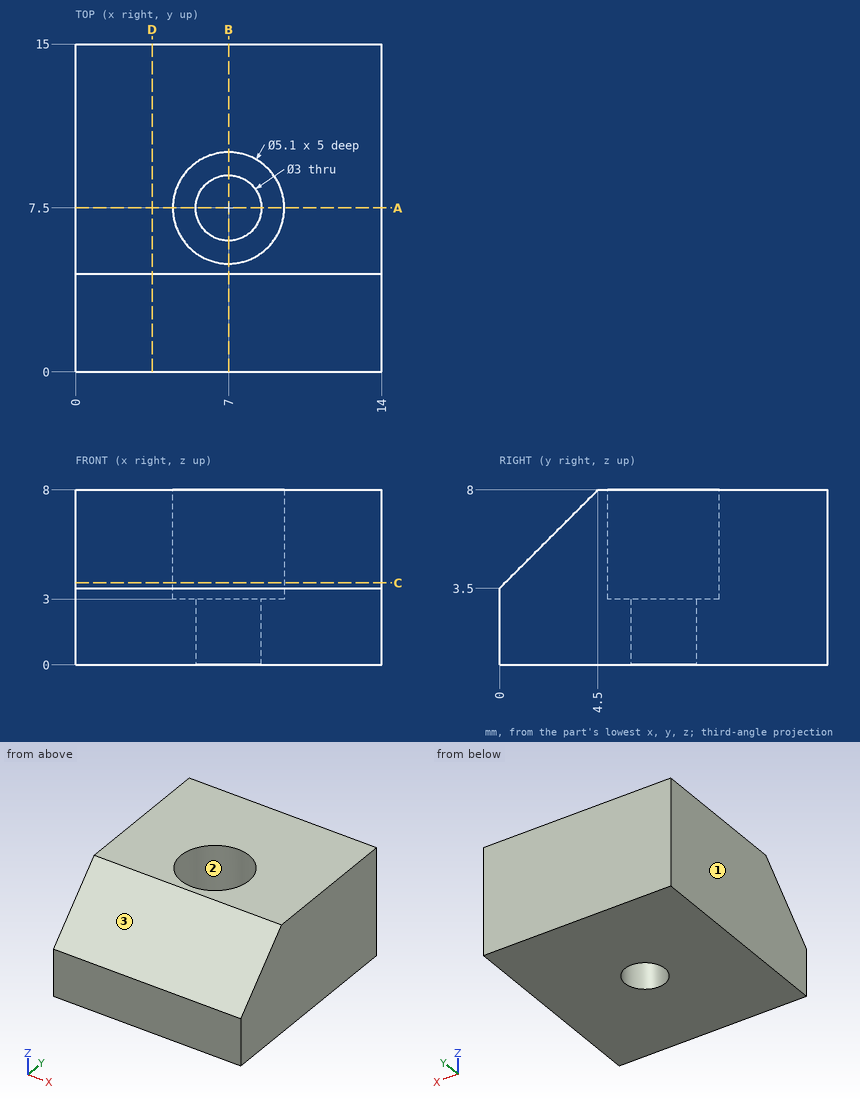
Source: three-view drawing plus pictorial views. Frame: mm from the lowest corner of the part. Coordinates: 2 decimals unless noted, no trailing zeros. Write each loop counter-clockwise with the first axis right and the second up, starting at its lowest first coordinate (ties: lowest second). Pieces come first, ordered by that corner, then holes. Notation, with made-up numbers: (-13, 11) -> (40, 11) arc R23 cw to (40, 27) -> close; hole circle Ø2 at (76.25, -23.75). An arc over 180 degrees is marked (long way). Answer as a JSON object with one key per item and string values.
1. Section C-C on z = 3.75. Return the cut outline in (x, y).
Result set:
{"outline": "(0, 0.25) -> (14, 0.25) -> (14, 15) -> (0, 15) -> close; hole circle Ø5.1 at (7, 7.5)"}
2. Section A-A on y = 7.5. Return the cut outline in (x, z).
Result set:
{"outline": "(0, 0) -> (5.5, 0) -> (5.5, 3) -> (4.45, 3) -> (4.45, 8) -> (0, 8) -> close; (8.5, 0) -> (14, 0) -> (14, 8) -> (9.55, 8) -> (9.55, 3) -> (8.5, 3) -> close"}
3. Section D-D on x = 3.5. Return the cut outline in (y, z), then the cut area to 3 significant figures.
Result set:
{"outline": "(0, 0) -> (15, 0) -> (15, 8) -> (4.5, 8) -> (0, 3.5) -> close", "area": "110 mm2"}
4. Section B-B on x = 7. Return the cut outline in (y, z), then the cut area to 3 significant figures.
Result set:
{"outline": "(0, 0) -> (6, 0) -> (6, 3) -> (4.95, 3) -> (4.95, 8) -> (4.5, 8) -> (0, 3.5) -> close; (9, 0) -> (15, 0) -> (15, 8) -> (10.05, 8) -> (10.05, 3) -> (9, 3) -> close", "area": "75.4 mm2"}
5. Mould query, pull axis X, two halves, no side actions, for the marked faces 1, 2 and 3. Classes: released by +X, released by -X, zero draft, split by the parting line, or undercut.
Result set:
{"face 1": "released by -X", "face 2": "undercut", "face 3": "zero draft"}
6. First-contact query: P1, Ø4, axis at x = 12, z = 5, coming from the -Y side; P2, Ø2.5, axis at x = 8, y = 7.5, coming from the +Z side. Flat tips, straight axial feed; report the tip coordinate or a pass-through.
Result set:
{"P1": "stops at y = 0", "P2": "stops at z = 3"}
7. Material intervals for line 1 (X direction, y = 7.5, z = 1.9); line 2 (Y direction, x = 7, z = 1.6); line 3 (X direction, y = 7.25, z = 6.25), sorted ascending. Write a range as from..to.
Result set:
{"line 1": "x = 0..5.5, 8.5..14", "line 2": "y = 0..6, 9..15", "line 3": "x = 0..4.46, 9.54..14"}
